CAD build for the part. Positions are in the model's coordinates, mm. A direction names the side the tool comes from. Coordinates: 2 decimals unless noted, no trailing zeros. Loops run counter-clockwise (first coordinate to the right, second up) from the corner with the lowest first, then second, coordinate; pieces in that order, holes last. Notation, with made-up numbers: (38, 31.25) -> (83, 31.25) arc R27 ccw to (83, 51.25) -> close; hole circle Ø5 at (-16.5, -23). An arc over 180 degrees is marked (long way). Return JSON: item names as keys, results as strings. Group by question number.
(1) Saw through at B-B on z = -0.5. Write the cut outline in (x, y).
(2) Tool access for faces 1 (the face through (-12, 1, -0.75)), 2 (the face through (-20, 2, 0)), 3 (the face through (-11.11, -3.084, 0.01)), 4 (the face through (-15, -3.5, 0)): list every direction of +Z, -Z, +X, -X, +Y, -Y with a clear straight run to the whole face (end or side of a thin tool).
(3) Probe L1, parallel to Y at x = 0, z = 0.3; L2, parallel to Y at x = -2.5, z = 0.15; L3, parallel to Y at x = -9.5, z = -0.55. List the from-to ranges inside material, lowest first.
(4) Saw through at D-D on x = -11. Write the cut outline in (y, z).
(5) Saw through at A-A on x = 0. Write the cut outline in (y, z).
(6) Saw through at C-C on x = -27.5. Write the cut outline in (y, z).
(7) Mould opens along X. For faces 5 (the face through (0, 4, 0)), 6 (the face through (-30.19, 0.15, 0.01)), 7 (the face through (-31.2, 3.66, 0.01)) say: pulls with the +X half, pulls with the -X half, needs draft (parallel to the pull), parting line crosses it, or undercut.
(8) Flat gauge pin, fed straight in: pin 1 Ø0.8 at (x, z) = (-14, 0) entering from -Y. Where does the tip first touch, or does it go through?
```python
from build123d import *

# Parameters (mm, degrees)
SKETCH1_R           = 1.5
BOSS_EXTRUDE1_DEPTH = 0.75
BOSS_EXTRUDE2_DEPTH = 0.75
FILLET1_R           = 1
FILLET2_R           = 0.5
FILLET3_R           = 1.5
CUT_REVOLVE1_ANGLE  = 90


with BuildPart() as part:
    # Sketch1 → Boss-Extrude1 (new, symmetric)
    with BuildSketch(Plane.XY):
        with BuildLine():
            Line((-13, 5.5), (-3.25, 5.5))
            Line((-3.25, 5.5), (-3.25, 4))
            Line((-3.25, 4), (3.25, 4))
            ThreePointArc((3.25, 4), (3.654082058, 0), (3.25, -4))
            Line((3.25, -4), (-8.75, -4))
            Line((-8.75, -4), (-13, 5.5))
        make_face()
        Circle(SKETCH1_R, mode=Mode.SUBTRACT)
    extrude(amount=BOSS_EXTRUDE1_DEPTH, both=True)

    # Sketch7 → Boss-Extrude2 (add, symmetric)
    with BuildSketch(Plane.XY):
        with BuildLine():
            Line((-13, 5.5), (-24, 5.5))
            ThreePointArc((-24, 5.5), (-31.29725976, 3.605342422), (-36.751078386, -1.6))
            Line((-36.751078386, -1.6), (-23.25, 2))
            Line((-23.25, 2), (-15.15, 2))
            Line((-15.15, 2), (-13.25, -2.1))
            Line((-13.25, -2.1), (-19.75, -1.5))
            Line((-19.75, -1.5), (-17.75, -3.5))
            Line((-17.75, -3.5), (-11.75, -3.5))
            Line((-11.75, -3.5), (-9.6, -2.1))
            Line((-9.6, -2.1), (-13, 5.5))
        make_face()
    extrude(amount=BOSS_EXTRUDE2_DEPTH, both=True)

    # Fillet1
    fillet1_edges = [part.edges().sort_by_distance(p)[0] for p in [
        (-9.6, -2.1, 0),
    ]]
    fillet(fillet1_edges, radius=FILLET1_R)

    # Fillet2
    fillet2_edges = [part.edges().sort_by_distance(p)[0] for p in [
        (-3.25, 4, 0),
        (3.25, 4, 0),
        (3.25, -4, 0),
        (-8.75, -4, 0),
        (-3.25, 5.5, 0),
        (-17.75, -3.5, 0),
        (-11.75, -3.5, 0),
    ]]
    fillet(fillet2_edges, radius=FILLET2_R)

    # Fillet3
    fillet3_edges = [part.edges().sort_by_distance(p)[0] for p in [
        (-23.25, 2, 0),
        (-15.15, 2, 0),
        (-13.25, -2.1, 0),
    ]]
    fillet(fillet3_edges, radius=FILLET3_R)

    # Sketch6 → Cut-Revolve1 (revolve, cut)
    with BuildSketch(Plane.XY.offset(0.75)):
        with BuildLine():
            Line((-27, 4.8), (-12, 4.8))
            ThreePointArc((-12, 4.8), (-19.5, 3.847375097), (-27, 4.8))
        make_face()
    revolve(axis=Axis((-27, 4.8, 0.75), (1, 0, 0)), revolution_arc=CUT_REVOLVE1_ANGLE, mode=Mode.SUBTRACT)


solid = part.part
```
Geometry results:
{
 "1": {"outline": "(-36.75, -1.6) -> (-23.44, 1.95) arc R1.5 cw to (-23.05, 2) -> (-16.11, 2) arc R1.5 cw to (-14.75, 1.13) -> (-14.35, 0.26) arc R1.5 cw to (-15.84, -1.86) -> (-19.75, -1.5) -> (-17.9, -3.35) arc R0.5 ccw to (-17.54, -3.5) -> (-11.9, -3.5) arc R0.5 ccw to (-11.63, -3.42) -> (-10.58, -2.74) arc R1 cw to (-9.12, -3.17) -> (-8.88, -3.7) arc R0.5 ccw to (-8.43, -4) -> (2.84, -4) arc R0.5 ccw to (3.33, -3.59) arc R20 ccw to (3.33, 3.59) arc R0.5 ccw to (2.84, 4) -> (-2.75, 4) arc R0.5 cw to (-3.25, 4.5) -> (-3.25, 5) arc R0.5 ccw to (-3.75, 5.5) -> (-24, 5.5) arc R15 ccw to start; hole circle Ø3 at (0, 0)"},
 "2": {"face 1": "-Z, +X, -X, +Y, -Y", "face 2": "+Z, -Z", "face 3": "+Z, -Z, -Y", "face 4": "+Z, -Z, -X, -Y"},
 "3": {"L1": "-4 to -1.5, 1.5 to 4", "L2": "-4 to 4", "L3": "-2.73 to 5.5"},
 "4": {"outline": "(-3.01, -0.75) -> (5.5, -0.75) -> (5.5, 0.75) -> (-3.01, 0.75) -> close"},
 "5": {"outline": "(-4, -0.75) -> (-1.5, -0.75) -> (-1.5, 0.75) -> (-4, 0.75) -> close; (1.5, -0.75) -> (4, -0.75) -> (4, 0.75) -> (1.5, 0.75) -> close"},
 "6": {"outline": "(0.87, -0.75) -> (5.09, -0.75) -> (5.09, 0.75) -> (0.87, 0.75) -> close"},
 "7": {"face 5": "needs draft", "face 6": "undercut", "face 7": "pulls with the -X half"},
 "8": {"pin 1": "y = -3.5"}
}
